Verification items for the finished model (mm, model axes). A direction names the side the tool comes from. Give positions to 0.01 mm unless a question says otherwise; leave off trailing zeros. Order: outer loops, then holes, each group sorted by start corner. A loop starts at its lowest first (then second) coordinate and runs counter-clockwise, first axis right, second up. Notation, with made-up numbers: M -14.5,34.5 L 8.5,34.5 A19 cw 8.5,50.5 Z; hole C -38,42.5 d2. An arc over 180 degrees is marked long. Answer as a JSON object with one key per item and string values.
Autodesk Inventor part; units mm, degrees
ref_plane "Start Plane" through (0, 0, 25.4) normal (0, 0, 1) x (1, 0, 0)
ref_plane "End Plane" through (0, 0, 50) normal (0, 0, 1) x (1, 0, 0)
ref_plane "Work Plane4" through (12.7, 0, 50) normal (0, 0.3827, 0.9239) x (1, 0, 0)
ref_plane "Start Plane" through (0, 0, 25.4) normal (0, 0, 1) x (1, 0, 0)
ref_plane "End Plane" through (0, 0, 50) normal (0, 0, 1) x (1, 0, 0)
sketch "Sketch" plane through (0, 0, 0) normal (0, 0, 1) x (1, 0, 0)
  line L0 (25.4, 0) -> (0, 0)
  line L1 (0, 0) -> (0, 25.4)
  line L2 (0, 25.4) -> (1.651, 25.4)
  line L3 (3.175, 23.876) -> (3.175, 6.477)
  line L4 (6.477, 3.175) -> (23.876, 3.175)
  line L5 (25.4, 1.651) -> (25.4, 0)
  line L6 (0, -11.0414) -> (0, 31.5385) construction
  line L7 (-11.0414, 0) -> (31.5385, 0) construction
  arc A0 (3.175, 6.477) -> (6.477, 3.175) centre (6.477, 6.477) ccw
  arc A1 (3.175, 23.876) -> (1.651, 25.4) centre (1.651, 23.876) ccw
  arc A2 (25.4, 1.651) -> (23.876, 3.175) centre (23.876, 1.651) ccw
  line L8 (0, 40.0545) -> (0, -19.5574) construction
  line L9 (-19.5574, 0) -> (40.0545, 0) construction
  point P0 (3.175, 25.4)
  point P1 (3.175, 3.175)
  point P2 (25.4, 3.175)
  dimension "d0" = 25.4
  dimension "d1" = 25.4
  dimension "d2" = 3.175
  dimension "d3" = 3.175
  dimension "d10" = 0
  dimension "d11" = 0
  dimension "d14" = 3.302
  dimension "d15" = 1.524
extrude "Body" add sketch "Sketch" along normal up to surface (24.6 mm away) from surface at 25.4
sketch "Sketch3" plane through (0, 0, 0) normal (0, 0, 1) x (1, 0, 0)
  line L0 (0, 0) -> (10, 0)
ref_plane "Work Plane3" through (0, 0, 0) normal (0, -1, 0) x (1, 0, 0)
ref_plane "Work Plane4" through (12.7, 0, 50) normal (0, 0.3827, 0.9239) x (1, 0, 0)
split "Split1" plane through (12.7, 0, 50) removes the side toward (0, 0.3827, 0.9239)
ref_plane "Work Plane5" through (0, 1058.349, 25.4) normal (0, 0, -1) x (-1, 0, 0)
split "Split2" plane through (0, 1058.349, 25.4) removes the side toward (0, 0, -1)
sketch "Sketch4" plane through (0, 0, 0) normal (0, -1, 0) x (1, 0, 0)
  line L0 (-2, 25.4) -> (12, 25.4)
  line L1 (-2, 50) -> (12, 50)
  dimension "d17" = 24.6
equation "\"d0\" = G_H"
equation "\"d1\" = G_H"
equation "\"d2\" = G_T"
equation "\"d3\" = G_T"
equation "\"d14\" = G_IR"
equation "\"d15\" = G_ER"
equation "\"d4\" = G_L"
equation "\"G_H\" = 25.4"
equation "\"G_T\" = 3.175"
equation "\"G_ER\" = 1.524"
equation "\"G_IR\" = 3.302"
equation "\"G_L\" = d17"
equation "\"ex\" = 0"
equation "\"G_OFFSET_START\" = -25.4"
equation "\"G_OFFSET_END\" = 0"
equation "\"d12\" = -G_OFFSET_START"
equation "\"d13\" = G_OFFSET_END + B_L"
equation "\"B_L\" = 50"
properties part number "AISC - L 1 x 1 x 1/8 - 0.969" material "Steel, Mild"
Q1. Material ranges on L1, parallel to Y at x = 11.25, z = 32.5 (3 decimals); L2, parallel to X at y = 6.25, z = 47; L3, parallel to Y at x = 4, z = 27.75, recorded low to high.
Resolved:
{"L1": "y = 0 to 3.175", "L2": "x = 0 to 3.18", "L3": "y = 0 to 4.29"}
Q2. Gauge pin test, flat ends, axial feed: pin 1 Ø4 at (y, z) = (20.5, 36.5) entering from +X (3 decimals); pin 2 Ø5 at (x, z) = (17.5, 33) entering from +Y (3 decimals). Record the tip position at first contact, or that the pin passes through.
Resolved:
{"pin 1": "stops at x = 3.175", "pin 2": "stops at y = 3.175"}
Q3. Tool access check on faces 1 (the face through (3, 5, 25.4)), 2 (the face through (3.175, 15, 34)). Record the directions out of +Z, -Z, +X, -X, +Y, -Y that give a thin tool (end or side, any length) a straight path to the whole face; none if there is none.
Resolved:
{"face 1": "-Z, +X, -X, +Y, -Y", "face 2": "+Z, -Z, +X, +Y"}
Q4. Section check B-B on x = 14.75. Record the cut outline in (y, z) (3 decimals), then the cut area to 3 significant figures.
Resolved:
{"outline": "M 0,25.4 L 3.175,25.4 L 3.175,48.685 L 0,50 Z", "area": "76.0 mm²"}
Q5. Section check C-C on y = 8.25. Record the cut outline in (x, z) (3 decimals).
Resolved:
{"outline": "M 0,25.4 L 3.175,25.4 L 3.175,46.583 L 0,46.583 Z"}
Q6. Section check D-D on z = 27.75. Record the cut outline in (x, y) (3 decimals), then the cut area to 3 significant figures.
Resolved:
{"outline": "M 0,0 L 25.4,0 L 25.4,1.651 A1.524 ccw 23.876,3.175 L 6.477,3.175 A3.302 cw 3.175,6.477 L 3.175,23.876 A1.524 ccw 1.651,25.4 L 0,25.4 Z", "area": "153 mm²"}
Q7. Section check A-A on z = 41. Record the cut outline in (x, y) (3 decimals), then the cut area to 3 significant figures.
Resolved:
{"outline": "M 0,0 L 25.4,0 L 25.4,1.651 A1.524 ccw 23.876,3.175 L 6.477,3.175 A3.302 cw 3.175,6.477 L 3.175,21.728 L 0,21.728 Z", "area": "141 mm²"}
